from build123d import *

# Parameters (mm, degrees)
F1_DEPTH = 10
F3_D     = 3.5


with BuildPart() as f1:
    # F0 (on Right) → F1 (new body)
    with BuildSketch(Plane.YZ):
        Polygon((-10, -3.070235), (10, -3.070235), (10, 2.929765), (-10, 2.929765), (-10, 1.429765), (0, 1.429765), (0, -1.570235), (-10, -1.570235), align=None)
    extrude(amount=F1_DEPTH)

    # F3 (through all)
    with Locations(Plane.XY.offset(2.929765)):
        with Locations((5, 5)):
            Hole(F3_D / 2)


solid = f1.part
Here's how the part is built. I have some questions about the finished solid (model axes, mm). A direction names the side the tool comes from. Give positions to 0.01 mm unless a question says otherwise; leave off trailing zeros. Loops run counter-clockwise (first coordinate to the right, second up) from the corner with the lowest first, then second, coordinate; pieces in that order, holes last. Notation, with made-up numbers: (-28.75, 51) -> (-11.75, 51) arc R17 ccw to (-11.75, 76) -> close; hole circle Ø10 at (83.5, 85). An arc over 180 degrees is marked (long way). Answer as a JSON object with one key per item and string values. Group by question number.
Item 1: I need wall thicknesses on L1, parallel to Z at x = 8.75, y = -1; L2, parallel to Y at x = 5, z = 0.55; L3, parallel to Y at x = 2.5, z = 0.15. Which ranges of each line are inside material? Lowest first, please.
Item 2: Imagine slicing it at B-B on y = -2.25. Write out the boundary of the cut face in (x, z).
Item 3: Will this pin go through, and if not, where does the flat tip stop? pin 1 (4 mm diameter, centred on x = 5, y = 5, fed in from +Z).
Item 4: On a 3-axis mill with a long thin cutter (end or side, diameter ignored), from which of +Z, -Z, +X, -X, +Y, -Y can I reach the whole of each face in a straight line? I mean faces 1 (the flat face through (5, -5, -1.57)), 2 (the flat face through (5, 10, 0)). Say none if no direction works.
Item 5: Imagine slicing it at A-A on x = 5. Write out the boundary of the cut face in (y, z).
Item 6: Imagine slicing it at C-C on z = -1. Write out the boundary of the cut face in (x, y), then the cut area to 3 significant figures.
Item 7: Imagine slicing it at D-D on x = 2.25. Write out the boundary of the cut face in (y, z), then the cut area to 3 significant figures.
Item 8: Thinking about a two-plate mould opening in Z: for faces 3 (the flat face through (5, -5, 1.43)), 4 (the flat face through (5, 0, 2.93)), 5 (the flat face through (10, 2, 0)), which applies, pulls with the +Z half, pulls with the -Z half, needs draft (parallel to the pull), parting line crosses it, or undercut?
Answer list:
{
 "1": {"L1": "z = -3.07 to -1.57, 1.43 to 2.93", "L2": "y = 0 to 3.25, 6.75 to 10", "L3": "y = 0 to 10"},
 "2": {"outline": "(0, -3.07) -> (10, -3.07) -> (10, -1.57) -> (0, -1.57) -> close; (0, 1.43) -> (10, 1.43) -> (10, 2.93) -> (0, 2.93) -> close"},
 "3": {"pin 1": "stops at z = 2.93"},
 "4": {"face 1": "+X, -X, -Y", "face 2": "+Z, -Z, +X, -X, +Y"},
 "5": {"outline": "(-10, -3.07) -> (3.25, -3.07) -> (3.25, 2.93) -> (-10, 2.93) -> (-10, 1.43) -> (0, 1.43) -> (0, -1.57) -> (-10, -1.57) -> close; (6.75, -3.07) -> (10, -3.07) -> (10, 2.93) -> (6.75, 2.93) -> close"},
 "6": {"outline": "(0, 0) -> (10, 0) -> (10, 10) -> (0, 10) -> close; hole circle Ø3.5 at (5, 5)", "area": "90.4 mm2"},
 "7": {"outline": "(-10, -3.07) -> (10, -3.07) -> (10, 2.93) -> (-10, 2.93) -> (-10, 1.43) -> (0, 1.43) -> (0, -1.57) -> (-10, -1.57) -> close", "area": "90.0 mm2"},
 "8": {"face 3": "undercut", "face 4": "pulls with the +Z half", "face 5": "needs draft"}
}
